Work out the finished part from the listing and answer in its coordinate system (mm). A direction names the side the tool comes from. Coordinates: 2 decimals unless noted, no trailing zeros. Write each loop counter-clockwise with the first axis right and the second up, starting at its lowest first coordinate (ties: lowest second). Pieces come first, ordered by that corner, then holes. Notation, with made-up numbers: (7.25, 53) - (19.25, 53) arc R28 ccw to (19.25, 71) - close; hole circle Ø5 at (-25, 39.25). An arc over 180 degrees is marked (long way). Use a Markdown table: item, result. Add a question column.
(1) Given pin 1 Ø4.5 at (x, z) = (9.525, -10.16) entering from -Y; pin 2 Ø3.5 at (x, z) = (19.05, -45.72) entering from -Y; pin 3 Ø2 at (x, z) = (19.05, -74.93) entering from -Y; pin 4 Ø3 at (x, z) = (28.58, -18.11) entering from +Y, each flat-ended and moving along its own axis, determine where each tip first touches the part or whether it passes through.
(2) For a pull along Z with two mould halves and no side action, classify faces 1 (the face through (18.29, 5.71, -44.73)), 2 (the face through (38.1, 5, -41)) as released by +Z, released by -Z, zero draft, split by the parting line, or undercut.
(3) The part is cut by section A-A, the plane x = 19.05. Give the vertices of the cut face in (y, z) (3 decimals).
(4) Find the intervals of material crossed by line 1 (X direction, y = 2.75, z = -10.16) (3 decimals); line 2 (X direction, y = 8.95, z = -10.16) (3 decimals); line 3 (X direction, y = 4.25, z = -45.72), in increasing order. Write a range as from..to.
(5) A tool of negligible diameter and unlimited length cuts with its end or side. For faces 3 (the face through (18, 1.999, -47)), 4 (the face through (27.355, 3.816, -10.431)), 5 (the face through (8.47, 8.54, -15.57)), from which of +Z, -Z, +X, -X, +Y, -Y can it reach the whole face along a straight path? Write none if from no direction.
(6) The part is cut by section D-D, the plane z = -59.69. Give the vertices of the cut face in (x, y) (3 decimals), then the cut area to 3 significant figures.
(7) The part is cut by section B-B, the plane z = -10.16. Give the vertices of the cut face in (x, y) (3 decimals), then the cut area to 3 significant figures.
(8) The part is cut by section C-C, the plane z = -45.72. Give the vertices of the cut face in (x, y) (3 decimals).
from build123d import *

# Parameters (mm, degrees)
SKETCH1_W           = 38.1
SKETCH1_H           = 82.55
BOSS_EXTRUDE1_DEPTH = 9.525
SKETCH2_R           = 2.77495
CUT_EXTRUDE1_DEPTH  = 1.99898
SKETCH3_R           = 1.25
CUT_EXTRUDE2_DEPTH  = 92.41574331
SKETCH4_R           = 2.74955
SKETCH4_R_2         = 2.77495
CUT_EXTRUDE3_DEPTH  = 1.99898
SKETCH5_R           = 1.25
CUT_EXTRUDE4_DEPTH  = 92.41574331
SKETCH6_R           = 2.75
CUT_EXTRUDE5_DEPTH  = 1.99898
SKETCH7_R           = 1.25
CUT_EXTRUDE6_DEPTH  = 10


with BuildPart() as part:
    # Sketch1 → Boss-Extrude1 (new body)
    with BuildSketch(Plane(origin=(0, 0, 0), x_dir=(1, 0, 0), z_dir=(0, 1, 0))):
        with Locations((19.05, 41.275)):
            Rectangle(SKETCH1_W, SKETCH1_H)
    extrude(amount=BOSS_EXTRUDE1_DEPTH)

    # Sketch2 → Cut-Extrude1 (cut)
    with BuildSketch(Plane.XZ):
        with Locations(Location((19.05, -74.93, 0), (0, 0, 270))):
            Circle(SKETCH2_R)
        with Locations(Location((19.05, -59.69, 0), (0, 0, 270))):
            Circle(SKETCH2_R)
    extrude(amount=-CUT_EXTRUDE1_DEPTH, mode=Mode.SUBTRACT)

    # Sketch3 → Cut-Extrude2 (cut, through all)
    with BuildSketch(Plane.XZ):
        with Locations(Location((19.05, -74.93, 0), (0, 0, 270))):
            Circle(SKETCH3_R)
        with Locations(Location((19.05, -59.69, 0), (0, 0, 270))):
            Circle(SKETCH3_R)
    extrude(amount=-CUT_EXTRUDE2_DEPTH, mode=Mode.SUBTRACT)

    # Sketch4 → Cut-Extrude3 (cut)
    with BuildSketch(Plane.XZ):
        with Locations(Location((19.05, -45.72, 0), (0, 0, 270))):
            Circle(SKETCH4_R)
        with Locations(Location((11.30403505, -45.72, 0), (0, 0, 270))):
            Circle(SKETCH4_R_2)
        with Locations(Location((26.79596495, -45.72, 0), (0, 0, 270))):
            Circle(SKETCH4_R_2)
    extrude(amount=-CUT_EXTRUDE3_DEPTH, mode=Mode.SUBTRACT)

    # Sketch5 → Cut-Extrude4 (cut, through all)
    with BuildSketch(Plane.XZ):
        with Locations(Location((19.05, -45.72, 0), (0, 0, 270))):
            Circle(SKETCH5_R)
        with Locations(Location((26.79596495, -45.72, 0), (0, 0, 270))):
            Circle(SKETCH5_R)
        with Locations(Location((11.30403505, -45.72, 0), (0, 0, 270))):
            Circle(SKETCH5_R)
    extrude(amount=-CUT_EXTRUDE4_DEPTH, mode=Mode.SUBTRACT)

    # Sketch6 → Cut-Extrude5 (cut)
    with BuildSketch(Plane(origin=(0, 9.525, 0), x_dir=(1, 0, 0), z_dir=(0, 1, 0))):
        with Locations(Location((9.525, 18.1102, 0), (0, 0, 270))):
            Circle(SKETCH6_R)
        with Locations(Location((9.525, 10.16, 0), (0, 0, 270))):
            Circle(SKETCH6_R)
        with Locations(Location((28.575, 18.1102, 0), (0, 0, 270))):
            Circle(SKETCH6_R)
        with Locations(Location((28.575, 10.16, 0), (0, 0, 270))):
            Circle(SKETCH6_R)
    extrude(amount=-CUT_EXTRUDE5_DEPTH, mode=Mode.SUBTRACT)

    # Sketch7 → Cut-Extrude6 (cut)
    with BuildSketch(Plane(origin=(0, 9.525, 0), x_dir=(1, 0, 0), z_dir=(0, 1, 0))):
        with Locations(Location((9.525, 18.1102, 0), (0, 0, 270))):
            Circle(SKETCH7_R)
        with Locations(Location((9.525, 10.16, 0), (0, 0, 270))):
            Circle(SKETCH7_R)
        with Locations(Location((28.575, 10.16, 0), (0, 0, 270))):
            Circle(SKETCH7_R)
        with Locations(Location((28.575, 18.1102, 0), (0, 0, 270))):
            Circle(SKETCH7_R)
    extrude(amount=-CUT_EXTRUDE6_DEPTH, mode=Mode.SUBTRACT)


solid = part.part
Model answer:
| question | item | result |
|---|---|---|
| 1 | pin 1 | y = 0 |
| 1 | pin 2 | y = 2 |
| 1 | pin 3 | through |
| 1 | pin 4 | y = 7.53 |
| 2 | face 1 | undercut |
| 2 | face 2 | zero draft |
| 3 | outline | (0, -82.55) - (9.525, -82.55) - (9.525, -76.18) - (1.999, -76.18) - (1.999, -77.705) - (0, -77.705) - close; (0, -72.155) - (1.999, -72.155) - (1.999, -73.68) - (9.525, -73.68) - (9.525, -60.94) - (1.999, -60.94) - (1.999, -62.465) - (0, -62.465) - close; (0, -56.915) - (1.999, -56.915) - (1.999, -58.44) - (9.525, -58.44) - (9.525, -46.97) - (1.999, -46.97) - (1.999, -48.47) - (0, -48.47) - close; (0, -42.97) - (1.999, -42.97) - (1.999, -44.47) - (9.525, -44.47) - (9.525, 0) - (0, 0) - close |
| 4 | line 1 | 0..8.275, 10.775..27.325, 29.825..38.1 |
| 4 | line 2 | 0..6.775, 12.275..25.825, 31.325..38.1 |
| 4 | line 3 | 0..10.05, 12.55..17.8, 20.3..25.55, 28.05..38.1 |
| 5 | face 3 | -Y |
| 5 | face 4 | +Y, -Y |
| 5 | face 5 | +Y |
| 6 | outline | (0, 0) - (16.275, 0) - (16.275, 1.999) - (17.8, 1.999) - (17.8, 9.525) - (0, 9.525) - close; (20.3, 1.999) - (21.825, 1.999) - (21.825, 0) - (38.1, 0) - (38.1, 9.525) - (20.3, 9.525) - close |
| 6 | area | 333 mm^2 |
| 7 | outline | (0, 0) - (8.275, 0) - (8.275, 7.526) - (6.775, 7.526) - (6.775, 9.525) - (0, 9.525) - close; (10.775, 0) - (27.325, 0) - (27.325, 7.526) - (25.825, 7.526) - (25.825, 9.525) - (12.275, 9.525) - (12.275, 7.526) - (10.775, 7.526) - close; (29.825, 0) - (38.1, 0) - (38.1, 9.525) - (31.325, 9.525) - (31.325, 7.526) - (29.825, 7.526) - close |
| 7 | area | 303 mm^2 |
| 8 | outline | (0, 0) - (8.529, 0) - (8.529, 1.999) - (10.054, 1.999) - (10.054, 9.525) - (0, 9.525) - close; (12.554, 1.999) - (14.079, 1.999) - (14.079, 0) - (16.3, 0) - (16.3, 1.999) - (17.8, 1.999) - (17.8, 9.525) - (12.554, 9.525) - close; (20.3, 1.999) - (21.8, 1.999) - (21.8, 0) - (24.021, 0) - (24.021, 1.999) - (25.546, 1.999) - (25.546, 9.525) - (20.3, 9.525) - close; (28.046, 1.999) - (29.571, 1.999) - (29.571, 0) - (38.1, 0) - (38.1, 9.525) - (28.046, 9.525) - close |
